CAD build for the part. Positions are in the model's coordinates, mm. A direction names the side the tool comes from. Give positions to 0.01 mm unless a question says otherwise; leave off trailing zeros. Order: outer loops, then holes, each group sorted by start corner. A loop starts at its lowest first (then second) coordinate and runs counter-clockwise, first axis right, second up.
Autodesk Inventor part; units mm, degrees
ref_plane "Начальная плоскость" through (0, 0, 65) normal (0, 0, 1) x (1, 0, 0)
ref_plane "Конечная плоскость" through (0, 0, 142.172) normal (0, 0, 1) x (1, 0, 0)
ref_plane "РабПлоскость8" through (0, -398.2295, 142.172) normal (0, 0, 1) x (1, 0, 0)
ref_plane "Начальная плоскость" through (0, 0, 65) normal (0, 0, 1) x (1, 0, 0)
ref_plane "Конечная плоскость" through (0, 0, 142.172) normal (0, 0, 1) x (1, 0, 0)
sketch "Эскиз" plane through (0, 0, 0) normal (0, 0, 1) x (1, 0, 0)
  line L0 (36, -32.5) -> (0, -32.5)
  line L1 (36, -32.5) -> (36, -28.696)
  line L2 (33.6994, -26.2039) -> (9.9215, -24.3017)
  line L3 (4.4, -18.3208) -> (4.4, 18.3208)
  line L4 (33.6994, 26.2039) -> (9.9215, 24.3017)
  line L5 (36, 28.696) -> (36, 32.5)
  line L6 (0, 32.5) -> (36, 32.5)
  line L7 (0, -32.5) -> (0, 32.5)
  arc A0 (4.4, -18.3208) -> (9.9215, -24.3017) centre (10.4, -18.3208) ccw
  arc A1 (9.9215, 24.3017) -> (4.4, 18.3208) centre (10.4, 18.3208) ccw
  arc A2 (36, -28.696) -> (33.6994, -26.2039) centre (33.5, -28.696) ccw
  arc A3 (33.6994, 26.2039) -> (36, 28.696) centre (33.5, 28.696) ccw
  line L8 (0, 45.5) -> (0, -45.5) construction
  line L9 (-7.2974, 0) -> (43.7847, 0) construction
  point P0 (36, -26.388)
  point P1 (4.4, -23.86)
  point P2 (4.4, 23.86)
  point P3 (36, 26.388)
  dimension "d3" = 36
  dimension "d5" = 4.4
  dimension "d7" = 65
  dimension "d9" = 8.64
  dimension "d11" = 8.64
  dimension "d13" = 6.112
  dimension "d15" = 6.112
  dimension "d22" = 6
  dimension "d23" = 2.5
  dimension "d24" = 32.5
  dimension "d25" = 0
extrude "Тело" add sketch "Эскиз" along normal up to surface (77.172 mm away) from surface at 65
sketch "Sketch3" plane through (0, 0, 0) normal (0, 0, 1) x (1, 0, 0)
  line L0 (0, 0) -> (10, 0)
ref_plane "Work Plane7" through (0, 0, 0) normal (0, -1, 0) x (1, 0, 0)
sketch "Sketch4" plane through (0, 0, 0) normal (0, -1, 0) x (1, 0, 0)
  line L0 (-2, 65) -> (12, 65)
  line L1 (-2, 142.172) -> (12, 142.172)
  dimension "d29" = 77.172
ref_plane "РабПлоскость8" through (0, -398.2295, 142.172) normal (0, 0, 1) x (1, 0, 0)
split "Разделение1" plane through (0, -398.2295, 142.172) removes the side toward (0, 0, 1)
ref_plane "РабПлоскость9" through (36, -398.2295, 65) normal (0, 0, -1) x (-1, 0, 0)
split "Разделение2" plane through (36, -398.2295, 65) removes the side toward (0, 0, -1)
equation "\"d3\" = b"
equation "\"d7\" = ParH"
equation "\"d22\" = R"
equation "\"d23\" = R1"
equation "\"d24\" = 0.5 * d7"
equation "\"d16\" = G_L"
equation "\"R1\" = 2.5"
equation "\"R\" = 6"
equation "\"t1\" = 4.4"
equation "\"t2\" = 7.2"
equation "\"ParH\" = 65"
equation "\"b\" = 36"
equation "\"msp_x1\" = 0.04 * b"
equation "\"msp_x2\" = -0.08 * t1 + 0.04 * b"
equation "\"G_L\" = d29"
equation "\"ex\" = 0"
equation "\"G_OFFSET_START\" = -65"
equation "\"G_OFFSET_END\" = -65"
equation "\"d26\" = -G_OFFSET_START"
equation "\"d27\" = G_OFFSET_END + B_L"
equation "\"B_L\" = 207.172"
properties part number "Швеллер 6.5U-77,17 ГОСТ 8240-97" material "Сталь, мягкая"
Item 1: Two-plate mould, pull along Y, no slides. Class faces 3 (the face through (6, -22.4, 103)), 4 (the face through (4.4, 0, 103)), 5 (the face through (36, -31, 103)), 6 (the face through (18, 32.5, 103)): released by +Y, released by -Y, zero draft, split by the parting line, or undercut.
Item 2: Slice it at D-D (y = 20). Give the cut face in (x, z).
Item 3: Wall check: L1, parallel to Y at x = 33.5, z = 131.5; L2, parallel to Y at x = 12, z = 75.5; L3, parallel to X at y = -13, z = 91.5. Give the ranges that are in metal, low to high.
Item 4: Drop a flat-ended pin along its axis: pin 1 Ø5 at (y, z) = (-3.5, 88.5) entering from +X. Give the stop position or say it passes through.
Item 5: Slice it at A-A (x = 22). Give the cut face in (y, z).
Item 6: Tool access for faces 1 (the face through (35.355, 27.019, 103.046)), 2 (the face through (3, 0, 65)): list every direction of +Z, -Z, +X, -X, +Y, -Y with a clear straight run to the whole face (end or side of a thin tool).
Item 7: Slice it at C-C (y = -10). Give the cut face in (x, z).
Item 8: Slice it at B-B (z = 126). Give the cut face in (x, y), and give its area (3 significant figures).
A:
1. face 3: undercut
1. face 4: undercut
1. face 5: zero draft
1. face 6: released by +Y
2. outline: (0, 65) - (4.64, 65) - (4.64, 142.17) - (0, 142.17) - close
3. L1: y = -32.5 to -26.19, 26.19 to 32.5
3. L2: y = -32.5 to -24.47, 24.47 to 32.5
3. L3: x = 0 to 4.4
4. pin 1: stops at x = 4.4
5. outline: (-32.5, 65) - (-25.27, 65) - (-25.27, 142.17) - (-32.5, 142.17) - close; (25.27, 65) - (32.5, 65) - (32.5, 142.17) - (25.27, 142.17) - close
6. face 1: +Z, -Z, +X
6. face 2: -Z, +X, -X, +Y, -Y
7. outline: (0, 65) - (4.4, 65) - (4.4, 142.17) - (0, 142.17) - close
8. outline: (0, -32.5) - (36, -32.5) - (36, -28.7) arc R2.5 ccw to (33.7, -26.2) - (9.92, -24.3) arc R6 cw to (4.4, -18.32) - (4.4, 18.32) arc R6 cw to (9.92, 24.3) - (33.7, 26.2) arc R2.5 ccw to (36, 28.7) - (36, 32.5) - (0, 32.5) - close
8. area: 763 mm2
